CAD build for the part. Positions are in the model's coordinates, mm. Face numbers are marked on the shaded views. A direction names the side the tool comes from. Round coordinates to 2 decimals unless told otherwise and drop trailing zeros. Order: outer loops, then holes, each group sorted by start corner. A loop starts at its lowest first (then second) coordinate and runs counter-clockwise, first axis right, second up. Notation, with made-up numbers: (69.25, 86) - (92.25, 86) arc R16 ccw to (92.25, 107) - close; hole circle Ø1 at (75, 45.25). An arc over 180 degrees is marked (long way). Use one line per item in the form item = value. Start each with the question number.
from build123d import *

# Parameters (mm, degrees)
SKETCH1_W                     = 5
SKETCH1_H                     = 5
BOSS_EXTRUDE1_DEPTH           = 10
HOLE_FOR_TUBING_R             = 1.1
CUT_EXTRUDE1_DEPTH            = 12.94095825
F_10_32_HOLE_FOR_LUER_SCREW_R = 2.0193
CUT_EXTRUDE2_DEPTH            = 4
F_4_40_SET_SCREW_HOLE_R       = 1.1303
CUT_EXTRUDE3_DEPTH            = 2
SKETCH2_W                     = 7.037684522
SKETCH2_H                     = 8.186757887
SKETCH2_W_2                   = 3.889087297
SKETCH2_H_2                   = 3.889087296
CUT_EXTRUDE4_DEPTH            = 5


with BuildPart() as part:
    # Sketch1 → Boss-Extrude1 (new body)
    with BuildSketch(Plane.XY):
        with Locations((-3.413043478, -0.260869565)):
            Rectangle(SKETCH1_W, SKETCH1_H)
    extrude(amount=BOSS_EXTRUDE1_DEPTH)

    # hole for tubing → Cut-Extrude1 (cut, through all)
    with BuildSketch(Plane(origin=(0, 0, 0), x_dir=(-1, 0, 0), z_dir=(0, 0, -1))):
        with Locations((3.413043478, -0.260869565)):
            Circle(HOLE_FOR_TUBING_R)
    extrude(amount=-CUT_EXTRUDE1_DEPTH, mode=Mode.SUBTRACT)

    # 10-32 hole for luer screw → Cut-Extrude2 (cut)
    with BuildSketch(Plane.XY.offset(10)):
        with Locations((-3.413043478, -0.260869565)):
            Circle(F_10_32_HOLE_FOR_LUER_SCREW_R)
    extrude(amount=-CUT_EXTRUDE2_DEPTH, mode=Mode.SUBTRACT)

    # 4-40 set screw hole → Cut-Extrude3 (cut)
    with BuildSketch(Plane(origin=(0, 2.239130435, 0), x_dir=(1, 0, 0), z_dir=(0, 1, 0))):
        with Locations(Location((-3.413043478, -2, 0), (0, 0, 180))):
            Circle(F_4_40_SET_SCREW_HOLE_R)
    extrude(amount=-CUT_EXTRUDE3_DEPTH, mode=Mode.SUBTRACT)

    # Sketch2 → Cut-Extrude4 (cut)
    with BuildSketch(Plane(origin=(0, 0, 0), x_dir=(-1, 0, 0), z_dir=(0, 0, -1))):
        with Locations((3.518842261, 0.133851948)):
            Rectangle(SKETCH2_W, SKETCH2_H)
        with Locations((3.413043479, -0.260869565)):
            Rectangle(SKETCH2_W_2, SKETCH2_H_2, mode=Mode.SUBTRACT)
    extrude(amount=-CUT_EXTRUDE4_DEPTH, mode=Mode.SUBTRACT)


solid = part.part
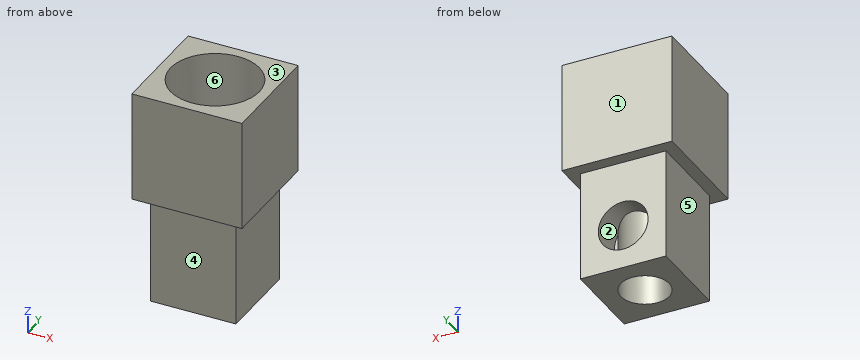
(1) Mould opens along Z. For the marked faces 1, 2 and 3 say: pulls with the +Z half, pulls with the -Z half, needs draft (parallel to the pull), parting line crosses it, or undercut.
(2) Flat gauge pins, fed straight in: P1, Ø1.2, axis at y = 0.5, z = 3, coming from the -X side; P2, Ø3, axis at y = -0.5, z = 3, coming from the +X side; P3, Ø1.2, axis at x = -2.5, y = -1, coming from the +Z side. Where does each tip first touch, or does it go through?
(3) Which spindle directions (+Z, -Z, +X, -X, +Y, -Y) get a long thin tool onto all of the face, cutting with end or side? Do the marked faces 4, 5 and 6. Say none if no direction does.
(4) Slice it at C-C (y = -0.85). Give the cut face in (x, z), and give its area (3 significant figures).
(5) Slice it at B-B (x = -2.6). Give the cut face in (y, z).
(6) Slice it at D-D (z = 5.5). Give the cut face in (x, y), and give its area (3 significant figures).
(7) Slice it at A-A (z = 2). Give the cut face in (x, y).
(8) Wall check: line 1 (X direction, y = 1.05, z = 2); line 2 (X direction, y = -0.85, z = 1); line 3 (Z direction, x = -1.9, y = -0.1). Give the ranges that are in metal, low to high. Write a range as [from, to].
Results list:
q1.face_1 = needs draft
q1.face_2 = undercut
q1.face_3 = pulls with the +Z half
q2.P1 = -5.36
q2.P2 = -1.47
q2.P3 = 6
q3.face_4 = -Z, +X, -X, -Y
q3.face_5 = -Z, -X, +Y, -Y
q3.face_6 = +Z
q4.outline = (-5.91, 5) - (-5.36, 5) - (-5.36, 0) - (-4.34, 0) - (-4.34, 6) - (-5.34, 6) - (-5.34, 10) - (-5.91, 10) - close; (-2.48, 0) - (-1.47, 0) - (-1.47, 5) - (-0.91, 5) - (-0.91, 10) - (-1.48, 10) - (-1.48, 6) - (-2.48, 6) - close
q4.area = 17.8 mm²
q5.outline = (-2.76, 5) - (-2.21, 5) - (-2.21, 0) - (-1, 0) - (-1, 6) - (-2.11, 6) - (-2.11, 10) - (-2.76, 10) - close; (0.48, 0) - (1.68, 0) - (1.68, 1.21) - (0.48, 1.21) - close; (0.48, 2.79) - (1.68, 2.79) - (1.68, 5) - (2.24, 5) - (2.24, 10) - (1.59, 10) - (1.59, 6) - (0.48, 6) - close
q6.outline = (-5.91, -2.76) - (-0.91, -2.76) - (-0.91, 2.24) - (-5.91, 2.24) - close; hole circle Ø2.2 at (-3.41, -0.26)
q6.area = 21.2 mm²
q7.outline = (-5.36, -2.21) - (-1.47, -2.21) - (-1.47, 1.68) - (-2.28, 1.68) - (-2.28, 0.24) - (-2.43, 0.24) arc R1.1 cw (long way) to (-4.39, 0.24) - (-4.54, 0.24) - (-4.54, 1.68) - (-5.36, 1.68) - close
q8.line_1 = [-5.36, -4.54], [-2.28, -1.47]
q8.line_2 = [-5.36, -4.34], [-2.48, -1.47]
q8.line_3 = [0, 6]
